```python
from build123d import *

# Parameters (mm, degrees)
F0_W     = 76.2
F0_H     = 63.5
F1_DEPTH = 25.4
F3_DEPTH = 50.8
F4_W     = 63.5
F4_H     = 21.465122
F5_DEPTH = 38.1


with BuildPart() as f1:
    # F0 (on Top) → F1 (new body)
    with BuildSketch(Plane.XY):
        with Locations((8.671692, -5.987014)):
            Rectangle(F0_W, F0_H)
    extrude(amount=F1_DEPTH)

    # F2 (on face) → F3 (join)
    with BuildSketch(Plane.XY.offset(25.4)):
        Polygon((-29.428308, -37.737014), (-13.991789, -37.737014), (-13.991789, 0.362986), (24.108211, 0.362986), (24.108211, 25.762986), (-29.428308, 25.762986), align=None)
    extrude(amount=F3_DEPTH)

    # F4 (on face) → F5 (join)
    with BuildSketch(Plane(origin=(-29.428308, 0, 0), x_dir=(0, -1, 0), z_dir=(-1, 0, 0))):
        with Locations((5.987014, 65.467439)):
            Rectangle(F4_W, F4_H)
    extrude(amount=F5_DEPTH)


solid = f1.part
```
Part model, mm, in its own coordinate system. A direction names the side the tool comes from. Round coordinates to 2 decimals unless told otherwise and drop trailing zeros. Loops run counter-clockwise (first coordinate to the right, second up) from the corner with the lowest first, then second, coordinate; pieces in that order, holes last. Notation, with made-up numbers: (-14, -5.5) -> (34, -5.5) arc R15 ccw to (34, 17.5) -> close; hole circle Ø10 at (6, 77). An arc over 180 degrees is marked (long way). Use CSV: the item, a comma, the result in double quotes. Start each with the question number.
1) Cut at C-C, the plane z = 61. Write the cut outline in (x, y).
2) Cut at D-D, the plane y = -2.5. Write the cut outline in (x, z), plus the area to 3 significant figures.
3) Drop flat-ended pins along their axis: P1, Ø11.5, axis at x = -46.5, y = -2.5, coming from the -Z side; P2, Ø20.5, axis at y = 13, z = 55.5, coming from the +X side; P3, Ø3, axis at x = 15.5, z = 48, coming from the -Y side. Give the stop position or say it passes through.
4) Cut at A-A, the plane y = 6.5. Write the cut outline in (x, z), plus the area to 3 significant figures.
5) Wall check: L1, parallel to Z at x = -54, y = -16; L2, parallel to X at y = -29, z = 56; L3, parallel to X at y = -5.5, z = 48.5. Give the ranges that are in metal, low to high. Write a range as [from, to].
6) Cut at B-B, the plane x = 22.5. Write the cut outline in (y, z), plus the area to 3 significant figures.
7) Which spindle directions (+Z, -Z, +X, -X, +Y, -Y) get a long thin tool onto all of the face, cutting with end or side? Do faces 1 (the flat face through (24.108, 13, 50)), 2 (the flat face through (-13.992, -19, 50)), 3 (the flat face through (-29.428, -6, 27)), 4 (the flat face through (-10, 25.763, 38)). Say none if no direction does.
Determined:
1,outline,"(-67.53, -37.74) -> (-13.99, -37.74) -> (-13.99, 0.36) -> (24.11, 0.36) -> (24.11, 25.76) -> (-67.53, 25.76) -> close"
2,outline,"(-67.53, 54.73) -> (-29.43, 54.73) -> (-29.43, 0) -> (46.77, 0) -> (46.77, 25.4) -> (-13.99, 25.4) -> (-13.99, 76.2) -> (-67.53, 76.2) -> close"
2,area,"3,540 mm2"
3,P1,"stops at z = 54.73"
3,P2,"stops at x = 24.11"
3,P3,"stops at y = 0.36"
4,outline,"(-67.53, 54.73) -> (-29.43, 54.73) -> (-29.43, 0) -> (46.77, 0) -> (46.77, 25.4) -> (24.11, 25.4) -> (24.11, 76.2) -> (-67.53, 76.2) -> close"
4,area,"5,470 mm2"
5,L1,"z = [54.73, 76.2]"
5,L2,"x = [-67.53, -13.99]"
5,L3,"x = [-29.43, -13.99]"
6,outline,"(-37.74, 0) -> (25.76, 0) -> (25.76, 76.2) -> (0.36, 76.2) -> (0.36, 25.4) -> (-37.74, 25.4) -> close"
6,area,"2,900 mm2"
7,face 1,"+Z, +X, +Y, -Y"
7,face 2,"+Z, +X, -Y"
7,face 3,"-Z, -X, +Y, -Y"
7,face 4,"+Z, -Z, +X, -X, +Y"
